Build history of the part. All positions in model axes, mm. Face numbers are marked on the shaded views. A direction names the side the tool comes from. Round coordinates to 2 decimals unless told otherwise and drop trailing zeros. Write each loop counter-clockwise with the first axis right and the second up, starting at its lowest first coordinate (ties: lowest second). Pieces come first, ordered by that corner, then holes. Notation, with made-up numbers: M -21,-37.5 L -1,-37.5 A10 cw -1,-33.5 Z; hole C 17,63.25 d8. An arc over 180 degrees is marked long. Use a Markdown table: item, result.
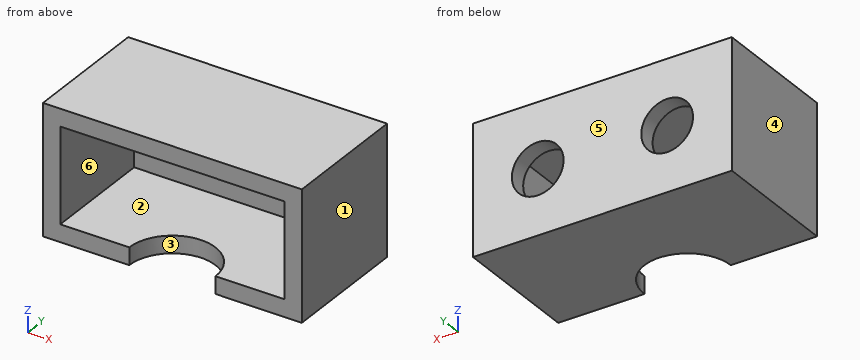
from build123d import *

# Parameters (mm, degrees)
SKETCH1_W           = 30
SKETCH1_H           = 15
BOSS_EXTRUDE1_DEPTH = 15
SKETCH2_W           = 26
SKETCH2_H           = 11
CUT_EXTRUDE1_DEPTH  = 13
SKETCH3_R           = 3
CUT_EXTRUDE2_DEPTH  = 13
SKETCH4_R           = 5
CUT_EXTRUDE3_DEPTH  = 5


with BuildPart() as part:
    # Sketch1 → Boss-Extrude1 (new body)
    with BuildSketch(Plane(origin=(0, 0, 0), x_dir=(1, 0, 0), z_dir=(0, 1, 0))):
        with Locations((15, 7.5)):
            Rectangle(SKETCH1_W, SKETCH1_H)
    extrude(amount=BOSS_EXTRUDE1_DEPTH)

    # Sketch2 → Cut-Extrude1 (cut)
    with BuildSketch(Plane.XZ):
        with Locations((15, -7.5)):
            Rectangle(SKETCH2_W, SKETCH2_H)
    extrude(amount=-CUT_EXTRUDE1_DEPTH, mode=Mode.SUBTRACT)

    # Sketch3 → Cut-Extrude2 (cut)
    with BuildSketch(Plane(origin=(0, 15, 0), x_dir=(1, 0, 0), z_dir=(0, 1, 0))):
        with Locations(Location((7.5, 7.5, 0), (0, 0, 270))):
            Circle(SKETCH3_R)
        with Locations(Location((22.5, 7.5, 0), (0, 0, 270))):
            Circle(SKETCH3_R)
    extrude(amount=-CUT_EXTRUDE2_DEPTH, mode=Mode.SUBTRACT)

    # Sketch4 → Cut-Extrude3 (cut)
    with BuildSketch(Plane(origin=(0, 0, -15), x_dir=(-1, 0, 0), z_dir=(0, 0, -1))):
        with Locations((-15, 0)):
            Circle(SKETCH4_R)
    extrude(amount=-CUT_EXTRUDE3_DEPTH, mode=Mode.SUBTRACT)


solid = part.part
Q1. Two-plate mould, pull along X, no slides. Class the marked faces 4, 5 and 6: +X half, -X half, draft (parallel to the pull), parting line (faces both ways), or undercut.
Response values:
| item | result |
|---|---|
| face 4 | -X half |
| face 5 | draft |
| face 6 | undercut |
Q2. Cut at D-D on z = -2.5. Give the cut face in (x, y), and give its area (3 significant figures).
Response values:
| item | result |
|---|---|
| outline | M 0,0 L 2,0 L 2,13 L 28,13 L 28,0 L 30,0 L 30,15 L 0,15 Z |
| area | 112 mm2 |
Q3. Drop a flat-ended pin along its axis: P1, Ø3.5, axis at x = 16.5, z = -9, coming from the -Y side. Give the stop position or say it passes through.
Response values:
| item | result |
|---|---|
| P1 | stops at y = 13 |
Q4. Drill centre lines: L1, parallel to X at y = 14.25, z = -7.5; L2, parallel to X at y = 4.75, z = -11.5; L3, parallel to Z at x = 13, y = 10.5. Where is each one in solid material? Low to high.
Response values:
| item | result |
|---|---|
| L1 | x = 0 to 4.5, 10.5 to 19.5, 25.5 to 30 |
| L2 | x = 0 to 2, 28 to 30 |
| L3 | z = -15 to -13, -2 to 0 |
Q5. Cut at C-C on x = 7. Give the cut face in (y, z), and give its area (3 significant figures).
Response values:
| item | result |
|---|---|
| outline | M 0,-15 L 15,-15 L 15,-10.46 L 13,-10.46 L 13,-13 L 0,-13 Z; M 0,-2 L 13,-2 L 13,-4.54 L 15,-4.54 L 15,0 L 0,0 Z |
| area | 70.2 mm2 |
Q6. Cut at B-B on z = -7.5. Give the cut face in (x, y), and give its area (3 significant figures).
Response values:
| item | result |
|---|---|
| outline | M 0,0 L 2,0 L 2,13 L 4.5,13 L 4.5,15 L 0,15 Z; M 10.5,13 L 19.5,13 L 19.5,15 L 10.5,15 Z; M 25.5,13 L 28,13 L 28,0 L 30,0 L 30,15 L 25.5,15 Z |
| area | 88.0 mm2 |
Q7. Cut at A-A on y = 11.25. Give the cut face in (x, z).
Response values:
| item | result |
|---|---|
| outline | M 0,-15 L 30,-15 L 30,0 L 0,0 Z; hole M 2,-13 L 28,-13 L 28,-2 L 2,-2 Z |
Q8. Which spindle directions (+Z, -Z, +X, -X, +Y, -Y) get a long thin tool onto all of the face, cutting with end or side? Do the marked faces 1, 2 and 3. Say none if no direction does.
Response values:
| item | result |
|---|---|
| face 1 | +Z, -Z, +X, +Y, -Y |
| face 2 | -Y |
| face 3 | -Z, -Y |
